The figure shows three views and two pictorial views of one solid part (mm, origin at its lowest corner). Answer the questions. A direction names the side the tool comes from. Coordinates: 2 decimals unless noted, no trailing zeros. Loops run counter-clockwise (first coordinate to the right, second up) from the corner with the lowest first, then second, coordinate; pieces in that order, holes last. Notation, with made-up numbers: (44, 35) - (101, 35) arc R20 cw to (101, 59) - close; hole circle Ø4 at (66, 40). An arc over 180 degrees is marked (long way). One line per question, with ' | ' between items.
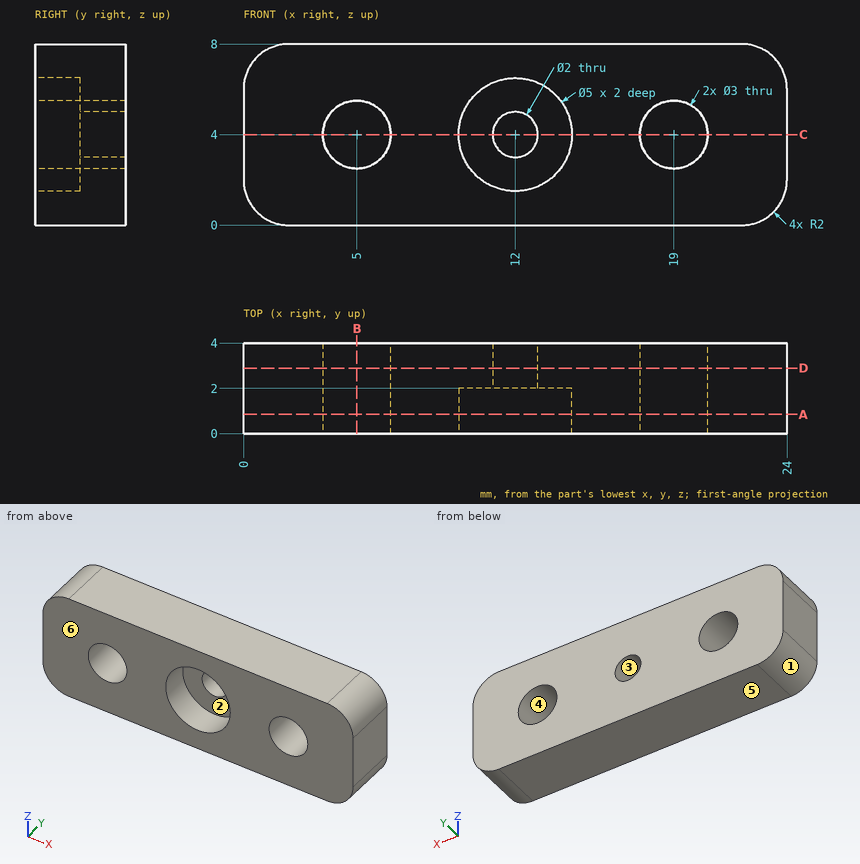
Item 1: The mould has two halves that part along Z. Classify the marked faces 3, 4, 5 and 6: pulls with the +Z half, pulls with the -Z half, needs draft (parallel to the pull), parting line crosses it, or undercut.
Taken from the geometry:
face 3: undercut | face 4: undercut | face 5: pulls with the -Z half | face 6: needs draft
Item 2: Find section B-B, the plane x = 5. Write down the section's boundary in (y, z).
Taken from the geometry:
outline: (0, 0) - (4, 0) - (4, 2.5) - (0, 2.5) - close; (0, 5.5) - (4, 5.5) - (4, 8) - (0, 8) - close
Item 3: Find section C-C, the plane z = 4. Write down the section's boundary in (x, y), plus the area to 3 significant figures.
Taken from the geometry:
outline: (0, 0) - (3.5, 0) - (3.5, 4) - (0, 4) - close; (6.5, 0) - (9.5, 0) - (9.5, 2) - (11, 2) - (11, 4) - (6.5, 4) - close; (13, 2) - (14.5, 2) - (14.5, 0) - (17.5, 0) - (17.5, 4) - (13, 4) - close; (20.5, 0) - (24, 0) - (24, 4) - (20.5, 4) - close | area: 58.0 mm2
Item 4: Find the intervals of material crossed by line 1 (X direction, y = 1.65, z = 4); line 2 (Z direction, x = 12, y = 1.3); line 3 (Z direction, x = 19, y = 1.75), in increasing order. Write a range as [from, to].
Taken from the geometry:
line 1: x = [0, 3.5], [6.5, 9.5], [14.5, 17.5], [20.5, 24] | line 2: z = [0, 1.5], [6.5, 8] | line 3: z = [0, 2.5], [5.5, 8]
Item 5: Find section A-A, the plane y = 0.85. Write down the section's boundary in (x, z).
Taken from the geometry:
outline: (0, 2) arc R2 ccw to (2, 0) - (22, 0) arc R2 ccw to (24, 2) - (24, 6) arc R2 ccw to (22, 8) - (2, 8) arc R2 ccw to (0, 6) - close; hole circle Ø3 at (5, 4); hole circle Ø5 at (12, 4); hole circle Ø3 at (19, 4)
Item 6: Find section D-D, the plane y = 2.9. Write down the section's boundary in (x, z), plus the area to 3 significant figures.
Taken from the geometry:
outline: (0, 2) arc R2 ccw to (2, 0) - (22, 0) arc R2 ccw to (24, 2) - (24, 6) arc R2 ccw to (22, 8) - (2, 8) arc R2 ccw to (0, 6) - close; hole circle Ø3 at (5, 4); hole circle Ø2 at (12, 4); hole circle Ø3 at (19, 4) | area: 171 mm2
Item 7: Which of the six approach directions +Z, -Z, +X, -X, +Y, -Y give full straight-line access (tool end or side, diameter ignored) to the marked faces 1 and 2?
Taken from the geometry:
face 1: -Z, -X, +Y, -Y | face 2: -Y
